Read the model definition and answer for the solid it produces. Units are mm, in the model's axes. Coordinates: 2 decimals unless noted, no trailing zeros. Order: outer loops, then holes, each group sorted by start corner. A loop starts at its lowest first (then second) coordinate and runs counter-clockwise, first axis right, second up. Notation, with made-up numbers: (25, 5.5) - (39, 5.5) arc R35 cw to (39, 42.5) - close; hole circle Ø10 at (54.5, 20). An arc over 180 degrees is marked (long way). Use one line per item in the form item = value. Start each with the question number.
Autodesk Inventor part; units mm, degrees
ref_plane "YZ Plane" through (0, 0, 0) normal (1, 0, 0) x (0, 1, 0)
ref_plane "XZ Plane" through (0, 0, 0) normal (0, 1, 0) x (-1, 0, 0)
ref_plane "XY Plane" through (0, 0, 0) normal (0, 0, 1) x (1, 0, 0)
sketch "Sketch1" plane through (0, 0, 0) normal (0, 0, 1) x (1, 0, 0)
  line L0 (0, 126.4897) -> (121.92, 126.4897)
  line L1 (121.92, 126.4897) -> (121.92, 29.9697)
  line L2 (121.92, 29.9697) -> (0, 29.9697)
  line L3 (0, 29.9697) -> (0, 126.4897)
  point P0 (0, 0)
  dimension "d0" = 96.52
  dimension "d1" = 121.92
extrude "Extrusion1" add sketch "Sketch1" along normal blind 2.54
fillet "Fillet1" radius 4.445 1 edges at (0, 126.4897, 1.27)
fillet "Fillet2" radius 4.445 1 edges at (121.92, 126.4897, 1.27)
sketch "Sketch2" plane through (0, 0, 2.54) normal (0, 0, 1) x (1, 0, 0)
  line L0 (56.642, 107.1857) -> (65.278, 107.1857)
  line L1 (65.278, 107.1857) -> (65.278, 98.5497)
  line L2 (65.278, 98.5497) -> (56.642, 98.5497)
  line L3 (56.642, 98.5497) -> (56.642, 107.1857)
  line L4 (121.92, 29.9697) -> (121.92, 122.0447)
  line L5 (0, 29.9697) -> (121.92, 29.9697)
  point P0 (0, 0)
  dimension "d6" = 8.636
  dimension "d7" = 8.636
  dimension "d8" = 56.642
  dimension "d9" = 68.58
extrude "Extrusion2" cut sketch "Sketch2" against normal blind 2.54
sketch "Sketch3" plane through (0, 0, 2.54) normal (0, 0, 1) x (1, 0, 0)
  line L0 (56.642, 98.5497) -> (56.642, 107.1857)
  line L1 (65.278, 107.1857) -> (65.278, 98.5497)
  line L2 (56.642, 107.1857) -> (65.278, 107.1857)
  point P0 (0, 0)
  point P1 (50.5968, 102.8677)
  point P2 (50.5968, 115.4407)
  point P3 (71.3232, 115.4407)
  point P4 (71.3232, 102.8677)
  dimension "d12" = 6.0452
  dimension "d13" = 6.0452
  dimension "d14" = 12.573
  dimension "d15" = 6.0452
  dimension "d16" = 6.0452
  dimension "d17" = 12.573
  dimension "d27" = 4.318
  dimension "d28" = 4.318
hole "Hole1" at (50.5968, 115.4407, 2.54) at (71.3232, 115.4407, 2.54) at (71.3232, 102.8677, 2.54) at (50.5968, 102.8677, 2.54) direction (0, 0, -1) diameter 2.0828 end through all
sketch "Sketch4" plane through (0, 0, 2.54) normal (0, 0, 1) x (1, 0, 0)
  line L0 (117.475, 126.4897) -> (4.445, 126.4897)
  line L1 (0, 122.0447) -> (0, 29.9697)
  line L2 (0, 29.9697) -> (121.92, 29.9697)
  point P0 (0, 0)
  point P1 (5.08, 121.4097)
  point P2 (5.08, 35.0497)
  dimension "d29" = 5.08
  dimension "d30" = 5.08
  dimension "d31" = 5.08
  dimension "d32" = 5.08
hole "Hole2" at (5.08, 121.4097, 2.54) at (5.08, 35.0497, 2.54) direction (0, 0, -1) diameter 2.6416 end through all
sketch "Sketch5" plane through (0, 0, 2.54) normal (0, 0, 1) x (1, 0, 0)
  line L0 (52.2478, 88.3389) -> (114.0206, 88.3389)
  line L1 (114.0206, 88.3389) -> (114.0206, 32.4589)
  line L2 (114.0206, 32.4589) -> (52.2478, 32.4589)
  line L3 (52.2478, 32.4589) -> (52.2478, 88.3389)
  line L4 (0, 29.9697) -> (121.92, 29.9697)
  line L5 (121.92, 29.9697) -> (121.92, 122.0447)
  point P0 (0, 0)
  point P1 (55.7022, 84.8845)
  point P2 (110.5662, 84.8845)
  point P3 (110.5662, 35.9133)
  point P4 (55.7022, 35.9133)
  dimension "d40" = 55.88
  dimension "d41" = 61.7728
  dimension "d42" = 3.4544
  dimension "d43" = 3.4544
  dimension "d44" = 3.4544
  dimension "d45" = 3.4544
  dimension "d46" = 3.4544
  dimension "d47" = 3.4544
  dimension "d48" = 3.4544
  dimension "d49" = 3.4544
  dimension "d50" = 2.4892
  dimension "d51" = 7.8994
hole "Hole3" at (55.7022, 84.8845, 2.54) at (110.5662, 84.8845, 2.54) at (110.5662, 35.9133, 2.54) at (55.7022, 35.9133, 2.54) direction (0, 0, -1) diameter 2.8448 end through all
sketch "Sketch6" plane through (121.92, 29.9697, 2.54) normal (1, 0, 0) x (0, 0, -1)
  line L0 (1.27, 57.15) -> (2.54, 57.15)
  line L1 (2.54, 57.15) -> (2.54, 31.75)
  line L2 (2.54, 31.75) -> (1.27, 31.75)
  line L3 (1.27, 31.75) -> (1.27, 57.15)
  line L4 (2.54, 0) -> (0, 0)
  line L5 (0, 0) -> (0, 92.075)
  point P0 (2.54, -29.9697)
  dimension "d59" = 25.4
  dimension "d60" = 31.75
  dimension "d61" = 1.27
  dimension "d62" = 1.27
extrude "Extrusion3" add sketch "Sketch6" along normal blind 1.27
properties part number "justlid"
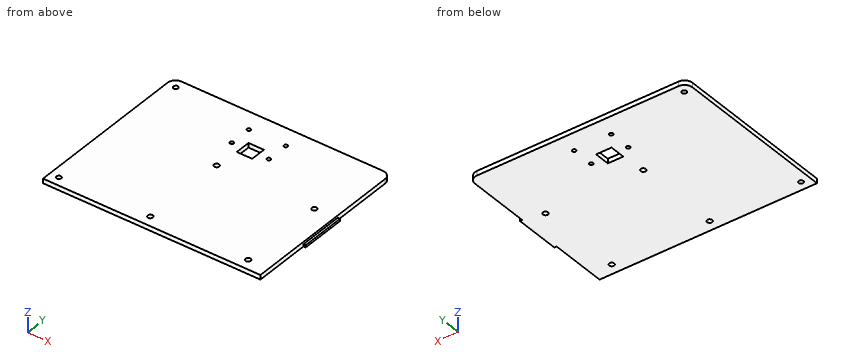
Q1. Consider probe 1 along Y at (x, z) = (57.5, 0.6); probe 2 along X at (y, z) = (106, 2.3); probe 3 along Y at (x, z) = (110, 0.5). Determine where each line is inside the solid, lowest interval first.
Q2. A cutting plane is placed at B-B (z = 0.4). Give the number of separate pieces and of enclosed holes in the cut face, then the cut area to 3 significant figures.
Q3. A cutting plane is placed at A-A (y = 100.5). Give the vertices of the cut face in (x, z).
Q4. Given P1, Ø1.7, axis at x = 71.32, y = 115.44, coming from the -Z side; P2, Ø3.5, axis at x = 110.57, y = 84.88, coming from the -Z side; P3, Ø0.6, axis at x = 123, z = 0.5, coming from the -Y side; P4, Ø0.6, axis at x = 122.5, y = 69, coming from the +Z side, each flat-ended and moving along its own axis, determine where each tip first touches the part or whether it passes through.
Result sheet:
q1.probe_1 = 29.97 to 98.55, 107.19 to 126.49
q1.probe_2 = 0 to 56.64, 65.28 to 121.92
q1.probe_3 = 29.97 to 34.61, 37.22 to 83.58, 86.19 to 126.49
q2.separate_pieces = 1
q2.enclosed_holes = 11
q2.area = 11,700 mm^2
q3.outline = (0, 0) - (56.64, 0) - (56.64, 2.54) - (0, 2.54) - close; (65.28, 0) - (121.92, 0) - (121.92, 2.54) - (65.28, 2.54) - close
q4.P1 = through
q4.P2 = 0
q4.P3 = 61.72
q4.P4 = 1.27
